Geometry: final body of the model. Coordinates: model frame, mm. Face numbers are marked on the shaded views. A direction names the side the tool comes from. Coordinates: 2 decimals unless noted, no trailing zeros. Order: outer loops, then holes, each group sorted by start corner. A loop starts at its lowest first (then second) coordinate and runs counter-clockwise, first axis right, second up. Notation, with made-up numbers: M 79,2 L 117,2 A37 cw 117,41 Z; hole C 12.25,-31 d11. An arc over 180 degrees is marked long. Use CSV: the item, a comma, the result in double quotes. Start each with the question number.
1. Section query A-A on x = 22. Return the cut outline in (y, z), and give its area (3 significant figures).
2. Set-up query: the marked faces 1, 2 and 3. Return all of +Z, -Z, +X, -X, +Y, -Y with unobstructed straight access to the full face (end or side cutting, diameter ignored); none if empty.
3. Section query C-C on x = -5. Return the cut outline in (y, z) (1 decimal).
4. Section query D-D on z = 1.75. State how many separate pieces and enclosed holes the cut face has, and give its area (3 significant figures).
5. First-contact query: P1, Ø12, axis at y = 67, z = 8, coming from the -X side; P2, Ø7.5, axis at x = 25.5, y = 66.5, coming from the +Z side; P3, Ø10, axis at x = -16, z = -6, coming from the +Y side. Flat tips, straight axial feed; report the tip coordinate or a pass-through.
6. Section query B-B on x = 34.5. Return the cut outline in (y, z).
7. Material intervals for line 1 (X direction, y = 8, z = 0) (3 decimals); line 2 (Y direction, x = 41, z = 8.5); line 3 (Y direction, x = 2.5, z = 7), sorted ascending.
8. Pull-direction query (X, two-part tool) for the marked faces 4, 5 and 6; classes: pulls with the +X half, pulls with the -X half, needs draft (parallel to the pull), parting line crosses it, or undercut.
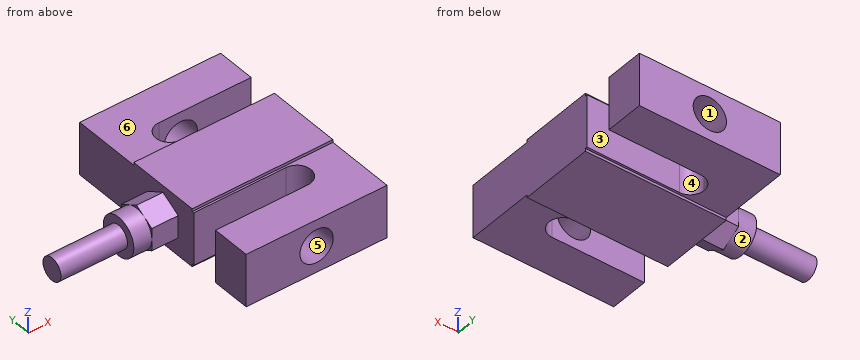
Autodesk Fusion 360 part; units mm, degrees
sketch "Sketch1" plane through (0, 0, 0) normal (0, 0, 1) x (1, 0, 0)
  line L0 (0, 0) -> (50.75, 0)
  line L1 (50.75, 0) -> (50.75, 52.25)
  line L2 (50.75, 52.25) -> (12.5, 52.25)
  line L3 (12.5, 52.25) -> (12.5, 62.25)
  line L4 (12.5, 62.25) -> (50.75, 62.25)
  line L5 (50.75, 62.25) -> (50.75, 76.25)
  line L6 (50.75, 76.25) -> (0, 76.25)
  line L7 (0, 76.25) -> (0, 24)
  line L8 (0, 24) -> (38.25, 24)
  line L9 (38.25, 24) -> (38.25, 14)
  line L10 (38.25, 14) -> (0, 14)
  line L11 (0, 14) -> (0, 0)
  line L12 (0, 24.75) -> (50.75, 24.75)
  line L13 (50.75, 51.5) -> (0, 51.5)
  dimension "d1" = 76.25
  dimension "d2" = 14
  dimension "d3" = 10
  dimension "d4" = 50.75
  dimension "d5" = 12.5
  dimension "d6" = 0.75
  dimension "d7" = 0.75
extrude "Extrude1" add sketch "Sketch1" along normal mid plane 19
extrude "Extrude2" add sketch "Sketch1" along normal mid plane 21 contours L1 L7 L12 L13
sketch "Sketch2" plane through (0, 0, 0) normal (-1, 0, 0) x (0, 0, 1)
  line L0 (9.5, 51.5) -> (9.5, 76.25)
  line L1 (9.5, 76.25) -> (-9.5, 76.25)
  line L2 (-9.5, 76.25) -> (-9.5, 51.5)
  line L3 (-9.5, 51.5) -> (-10.5, 51.5)
  line L4 (-10.5, 51.5) -> (-10.5, 24.75)
  line L5 (-10.5, 24.75) -> (-9.5, 24.75)
  line L6 (-9.5, 24.75) -> (-9.5, 24)
  line L7 (-9.5, 24) -> (9.5, 24)
  line L8 (9.5, 24) -> (9.5, 24.75)
  line L9 (9.5, 24.75) -> (10.5, 24.75)
  line L10 (10.5, 24.75) -> (10.5, 51.5)
  line L11 (10.5, 51.5) -> (9.5, 51.5)
  line L12 (8.0829, 38.125) -> (4.0415, 45.125)
  line L13 (4.0415, 45.125) -> (-4.0415, 45.125)
  line L14 (-4.0415, 45.125) -> (-8.0829, 38.125)
  line L15 (-8.0829, 38.125) -> (-4.0415, 31.125)
  line L16 (-4.0415, 31.125) -> (4.0415, 31.125)
  line L17 (4.0415, 31.125) -> (8.0829, 38.125)
  line L18 (-9.5, 0) -> (9.5, 0)
  line L19 (0, 76.25) -> (0, 24)
  circle A0 centre (0, 38.125) radius 4.1
  circle A1 centre (0, 38.125) radius 7
  point P0 (0, 38.125)
  dimension "d12" = 7
  dimension "d13" = 38.125
  dimension "d14" = 8.2
  dimension "d15" = 14
extrude "Extrude3" add sketch "Sketch2" along normal blind 9.5 contours L13 L14 A1 | L19 A0 A1 | L12 L13 A1 | L19 A0 A1 | L19 A0 | L19 A0 | L12 L17 A1 | L14 L15 A1 | L15 L16 A1 | L16 L17 A1
extrude "Extrude4" add sketch "Sketch2" along normal blind 16 contours L19 A0 A1 | L19 A0 A1 | L19 A0 | L19 A0
extrude "Extrude5" add sketch "Sketch2" along normal blind 40 contours L19 A0 | L19 A0
fillet "Fillet1" radius 5 4 edges at (38.25, 14, 0) (38.25, 24, 0) (12.5, 62.25, 0) (12.5, 52.25, 0)
sketch "Sketch3" plane through (0, 76.25, 0) normal (0, 1, 0) x (-1, 0, 0)
  line L0 (0, -9.5) -> (0, 9.5)
  line L1 (0, 9.5) -> (-50.75, 9.5)
  line L2 (-50.75, 9.5) -> (-50.75, -9.5)
  line L3 (-50.75, -9.5) -> (0, -9.5)
  circle A0 centre (-25.375, 0) radius 6
  line L4 (0, 4.0415) -> (0, -4.0415)
  line L5 (-50.75, 0) -> (0, 0)
  dimension "d24" = 25.375
  dimension "d25" = 12
extrude "Extrude6" cut sketch "Sketch3" against normal up to surface (14 mm away) contours A0 L5 | A0 L5
extrude "Extrude7" cut sketch "Sketch3" along normal up to surface (14 mm away) from surface at -76.25 contours A0 L5 | A0 L5
thread "Thread1"
thread "Thread2"
equation "d8 = ( 19 / 2 ) * 1 mm"
equation "d10 = ( 21 / 2 ) * 1 mm"
equation "d12 = ( 14 / 2 ) * 1 mm"
equation "d13 = d1 / 2"
equation "d24 = d4 / 2"
Results list:
1,outline,"M 0,-9.5 L 14,-9.5 L 14,-4.96 L 0,-4.96 Z; M 0,4.96 L 14,4.96 L 14,9.5 L 0,9.5 Z; M 24,-9.5 L 24.75,-9.5 L 24.75,-10.5 L 51.5,-10.5 L 51.5,-9.5 L 52.25,-9.5 L 52.25,9.5 L 51.5,9.5 L 51.5,10.5 L 24.75,10.5 L 24.75,9.5 L 24,9.5 Z; M 62.25,-9.5 L 76.25,-9.5 L 76.25,-4.96 L 62.25,-4.96 Z; M 62.25,4.96 L 76.25,4.96 L 76.25,9.5 L 62.25,9.5 Z"
1,area,"844 mm²"
2,face 1,"+Y"
2,face 2,"-X"
2,face 3,"+Z, -Z, +X"
3,outline,"M 31.1,-4 L 38.1,-8.1 L 45.1,-4 L 45.1,4 L 38.1,8.1 L 31.1,4 Z"
4,separate pieces,"3"
4,enclosed holes,"0"
4,area,"3,200 mm²"
5,P1,"stops at x = 0"
5,P2,"stops at z = 9.5"
5,P3,"stops at y = 45.05"
6,outline,"M 0,-9.5 L 14.16,-9.5 L 14.16,9.5 L 0,9.5 Z; M 23.84,-9.5 L 24.75,-9.5 L 24.75,-10.5 L 51.5,-10.5 L 51.5,-9.5 L 52.25,-9.5 L 52.25,9.5 L 51.5,9.5 L 51.5,10.5 L 24.75,10.5 L 24.75,9.5 L 23.84,9.5 Z; M 62.25,-9.5 L 76.25,-9.5 L 76.25,9.5 L 62.25,9.5 Z"
7,line 1,"x = 0 to 19.375, 31.375 to 50.75"
7,line 2,"y = 0 to 52.25, 62.25 to 76.25"
7,line 3,"y = 0 to 14, 24 to 76.25"
8,face 4,"pulls with the +X half"
8,face 5,"undercut"
8,face 6,"needs draft"
